Part print with two shaded views. Sizes in mm from the minimum x, y, z corner. A direction names the side the tool comes from. Round coordinates to 2 decimals unless told otherwise and drop trailing zeros. Loops run counter-clockwise (first coordinate to the right, second up) from the corner with the lowest first, then second, coordinate; pieces in that order, holes last. Notation, with made-up numbers: (-11, 30) - (47, 30) arc R23 cw to (47, 48) - close; hole circle Ø8 at (4, -21.5). An arc over 180 degrees is marked (long way). Use a Markdown table: item, result.
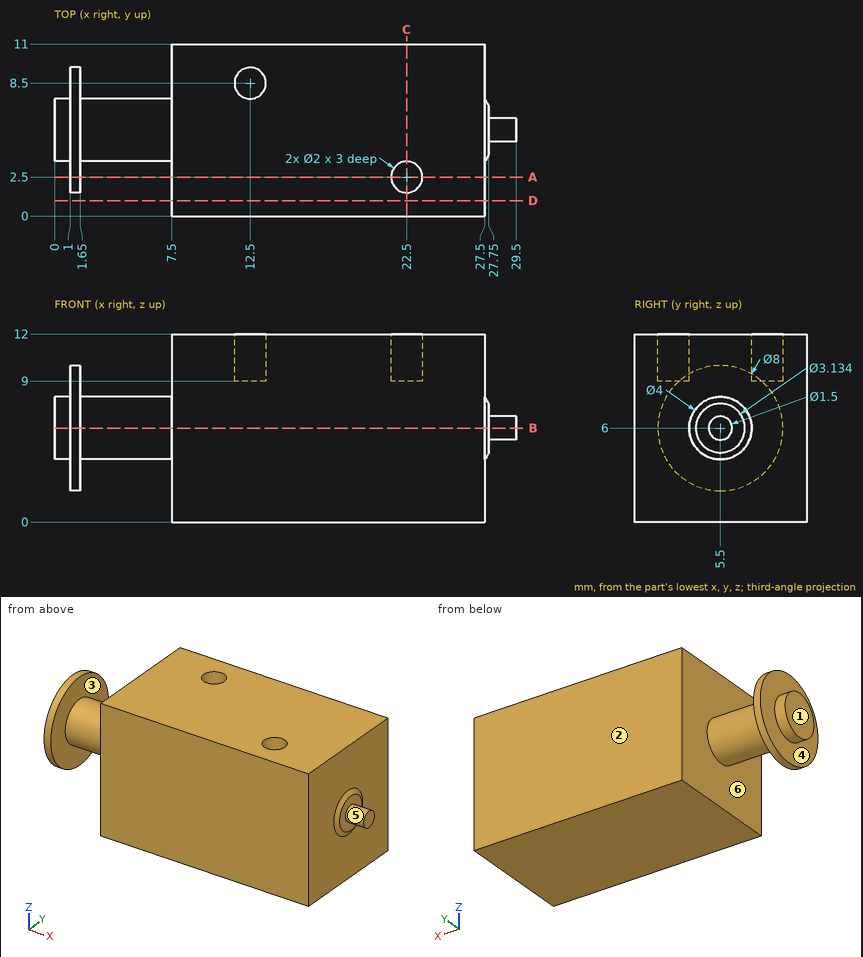
Q1. Cut at A-A, the plane y = 2.5. List the corners of the cut face in (x, z), plus the area to 3 significant figures.
Results found:
| item | result |
|---|---|
| outline | (1, 3.35) - (1.65, 3.35) - (1.65, 8.65) - (1, 8.65) - close; (7.5, 0) - (27.5, 0) - (27.5, 12) - (23.5, 12) - (23.5, 9) - (21.5, 9) - (21.5, 12) - (7.5, 12) - close |
| area | 237 mm2 |
Q2. Which spindle directions (+Z, -Z, +X, -X, +Y, -Y) get a long thin tool onto all of the face, cutting with end or side? Do the marked faces 4, 5 and 6. Say none if no direction does.
Results found:
| item | result |
|---|---|
| face 4 | -X |
| face 5 | +X |
| face 6 | none |
Q3. Cut at C-C, the plane x = 22.5. List the corners of the cut face in (y, z), plus the area to 3 significant figures.
Results found:
| item | result |
|---|---|
| outline | (0, 0) - (11, 0) - (11, 12) - (3.5, 12) - (3.5, 9) - (1.5, 9) - (1.5, 12) - (0, 12) - close |
| area | 126 mm2 |
Q4. Pull direction X, two halves, no side cores. Call the marked faces 1, 2 and 3: pulls with the +X half, pulls with the -X half, needs draft (parallel to the pull), parting line crosses it, or undercut.
Results found:
| item | result |
|---|---|
| face 1 | pulls with the -X half |
| face 2 | needs draft |
| face 3 | undercut |
Q5. Cut at D-D, the plane y = 1. List the corners of the cut face in (x, z), plus the area to 3 significant figures.
Results found:
| item | result |
|---|---|
| outline | (7.5, 0) - (27.5, 0) - (27.5, 12) - (7.5, 12) - close |
| area | 240 mm2 |
Q6. Cut at B-B, the plane z = 6. List the corners of the cut face in (x, y), plus the area to 3 significant figures.
Results found:
| item | result |
|---|---|
| outline | (0, 3.5) - (1, 3.5) - (1, 1.5) - (1.65, 1.5) - (1.65, 3.5) - (7.5, 3.5) - (7.5, 0) - (27.5, 0) - (27.5, 3.5) - (27.75, 3.93) - (27.75, 4.75) - (29.5, 4.75) - (29.5, 6.25) - (27.75, 6.25) - (27.75, 7.07) - (27.5, 7.5) - (27.5, 11) - (7.5, 11) - (7.5, 7.5) - (1.65, 7.5) - (1.65, 9.5) - (1, 9.5) - (1, 7.5) - (0, 7.5) - close |
| area | 256 mm2 |
Q7. Drop flat-ended pins along their axis: pin 1 (6 mm diameter, centred on y = 2.5, z = 3.5, fed in from +X); pin 2 (5 mm diameter, centred on x = 18.5, z = 7, fed in from -Y); pin 3 (1.6 mm diameter, centred on x = 12.5, y = 8.5, fed in from +Z); pin 4 (1 mm diameter, centred on y = 3.5, z = 9, fed in from -X). Give the stop position or say it passes through.
Results found:
| item | result |
|---|---|
| pin 1 | stops at x = 27.75 |
| pin 2 | stops at y = 0 |
| pin 3 | stops at z = 9 |
| pin 4 | stops at x = 1 |
Q8. Probe line 1 (X direction, y = 2.25, z = 6); line 2 (Y direction, x = 12.5, z = 11.3); line 3 (Y direction, x = 22.5, z = 10.8). List the from-to ranges inside material, lowest first.
Results found:
| item | result |
|---|---|
| line 1 | x = 1 to 1.65, 7.5 to 27.5 |
| line 2 | y = 0 to 7.5, 9.5 to 11 |
| line 3 | y = 0 to 1.5, 3.5 to 11 |
